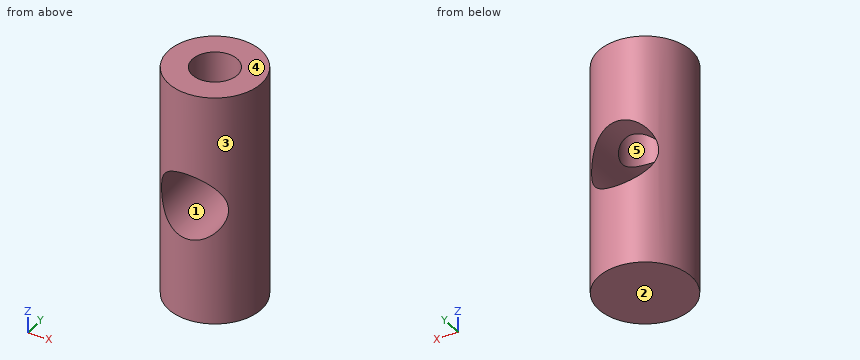
from build123d import *

# Parameters (mm, degrees)
ESQUISSE1_R                  = 7
BOSS_EXTRU_1_DEPTH           = 17.5
ENL_V_MAT_EXTRU_1_DEPTH      = 21.105969263
ENL_V_MAT_EXTRU_1_DEPTH_BACK = 21.105969263
ESQUISSE2_R                  = 5
TROU_TARAUD_M81_D            = 6.8
TROU_TARAUD_M81_DEPTH        = 20
TROU_TARAUD_M81_TIP          = 2.042926105


with BuildPart() as part:
    # Esquisse1 → Boss.-Extru.1 (new, symmetric)
    with BuildSketch(Plane.XY):
        Circle(ESQUISSE1_R)
    extrude(amount=BOSS_EXTRU_1_DEPTH, both=True)

    # Esquisse2 → Enlèv. mat.-Extru.1 (cut, two sides: drawn at the far end of the back side and taken through both)
    with BuildSketch(Plane(origin=(0, 0, 0), x_dir=(1, 0, 0), z_dir=(0, 1, 0)).offset(-ENL_V_MAT_EXTRU_1_DEPTH_BACK)):
        with Locations(Location((0, 0, 0), (0, 0, 270))):
            Circle(ESQUISSE2_R)
    extrude(amount=ENL_V_MAT_EXTRU_1_DEPTH + ENL_V_MAT_EXTRU_1_DEPTH_BACK, mode=Mode.SUBTRACT)

    # Trou taraudé M81
    with Locations(Plane.XY.offset(17.5)):
        with Locations((0, 0)):
            Hole(TROU_TARAUD_M81_D / 2, depth=TROU_TARAUD_M81_DEPTH)
            with Locations((0, 0, -(TROU_TARAUD_M81_DEPTH + TROU_TARAUD_M81_TIP / 2))):  # 118° drill point
                Cone(0, TROU_TARAUD_M81_D / 2, TROU_TARAUD_M81_TIP, mode=Mode.SUBTRACT)


solid = part.part
Input: part model. Units: mm. Frame: model coordinates. Face numbers are marked on the shaded views. A direction names the side the tool comes from. Give positions to 0.01 mm unless a question says otherwise; leave off trailing zeros. Order: outer loops, then holes, each group sorted by start corner. A loop starts at its lowest first (then second) coordinate and runs counter-clockwise, first axis right, second up.
Q1. Set-up query: the marked faces 4 and 5. Return all of +Z, -Z, +X, -X, +Y, -Y with unobstructed straight access to the full face (end or side cutting, diameter ignored); none if empty.
Checked values:
face 4: +Z, +X, -X, +Y, -Y
face 5: +Z
Q2. Section C-C on y = -5.5. Output: boundary loops of the cut face in (x, z).
Checked values:
outline: (-4.33, -17.5) - (4.33, -17.5) - (4.33, -2.5) arc R5 cw to (-4.33, -2.5) - close; (-4.33, 2.5) arc R5 cw to (4.33, 2.5) - (4.33, 17.5) - (-4.33, 17.5) - close
Q3. Draft query along X for the marked faces 1, 2 and 3. Return one class per face: +X half, -X half, draft (parallel to the pull), parting line (faces both ways), or undercut.
Checked values:
face 1: undercut
face 2: draft
face 3: parting line
Q4. Section A-A on x = 0. Output: boundary loops of the cut face in (y, z).
Checked values:
outline: (-7, -17.5) - (7, -17.5) - (7, -5) - (-7, -5) - close; (-7, 5) - (-3.4, 5) - (-3.4, 17.5) - (-7, 17.5) - close; (3.4, 5) - (7, 5) - (7, 17.5) - (3.4, 17.5) - close
Q5. Ray query, probe 1 along Y at (x, z) = (0, 14.75); probe 2 along Z at (x, y) = (0, 0.5); probe 3 along X at (y, z) = (-2.5, -2). Return the intervals inside material, ascending.
Checked values:
probe 1: y = -7 to -3.4, 3.4 to 7
probe 2: z = -17.5 to -5
probe 3: x = -6.54 to -4.58, 4.58 to 6.54
Q6. Contact query for flat-ended pins moving along their axis: pin 1 Ø2 at (y, z) = (-4, 6.5) entering from -X; pin 2 Ø5 at (x, z) = (5, 9) entering from +Y; pin 3 Ø2 at (x, z) = (-4.5, 3) entering from +Y. Output: stop coordinate, or through.
Checked values:
pin 1: stops at x = -6.32
pin 2: stops at y = 6.54
pin 3: stops at y = 6
Q7. Section B-B on y = 0. Output: boundary loops of the cut face in (x, z), and give its area (3 significant figures).
Checked values:
outline: (-7, -17.5) - (7, -17.5) - (7, 17.5) - (3.4, 17.5) - (3.4, 3.67) arc R5 cw (long way) to (-3.4, 3.67) - (-3.4, 17.5) - (-7, 17.5) - close
area: 324 mm2
Q8. Section D-D on z = 3. Output: boundary loops of the cut face in (x, y).
Checked values:
outline: (-4, -5.74) - (-4, 5.74) arc R7 ccw to start; (4, -5.74) arc R7 ccw to (4, 5.74) - close
